Part model, mm, in its own coordinate system. Face numbers are marked on the shaded views. Round coordinates to 2 decimals unless told otherwise and drop trailing zeros. Put each result on its own line as item: value.
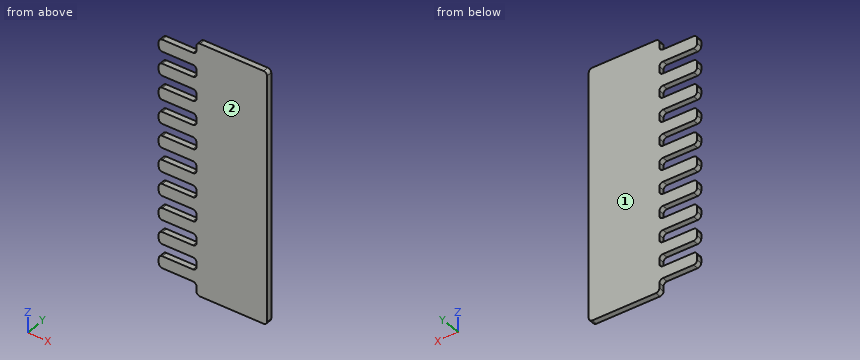
from build123d import *

# Parameters (mm, degrees)
BOSS_EXTRUDE1_DEPTH = 1.2


with BuildPart() as part:
    # Sketch1 → Boss-Extrude1 (new body)
    with BuildSketch(Plane(origin=(0, 0, 0), x_dir=(1, 0, 0), z_dir=(0, 1, 0))):
        with BuildLine():
            Line((-0.75, 2.54), (-7.25, 2.54))
            ThreePointArc((-7.25, 2.54), (-7.780330086, 2.759669914), (-8, 3.29))
            Line((-8, 3.29), (-8, 4.33))
            ThreePointArc((-8, 4.33), (-7.780330086, 4.860330086), (-7.25, 5.08))
            Line((-7.25, 5.08), (-0.75, 5.08))
            ThreePointArc((-0.75, 5.08), (-0.219669914, 5.299669914), (0, 5.83))
            Line((0, 5.83), (0, 6.87))
            ThreePointArc((0, 6.87), (-0.219669914, 7.400330086), (-0.75, 7.62))
            Line((-0.75, 7.62), (-7.25, 7.62))
            ThreePointArc((-7.25, 7.62), (-7.780330086, 7.839669914), (-8, 8.37))
            Line((-8, 8.37), (-8, 9.41))
            ThreePointArc((-8, 9.41), (-7.780330086, 9.940330086), (-7.25, 10.16))
            Line((-7.25, 10.16), (-0.75, 10.16))
            ThreePointArc((-0.75, 10.16), (-0.219669914, 10.379669914), (0, 10.91))
            Line((0, 10.91), (0, 11.95))
            ThreePointArc((0, 11.95), (-0.219669914, 12.480330086), (-0.75, 12.7))
            Line((-0.75, 12.7), (-7.25, 12.7))
            ThreePointArc((-7.25, 12.7), (-7.780330086, 12.919669914), (-8, 13.45))
            Line((-8, 13.45), (-8, 14.49))
            ThreePointArc((-8, 14.49), (-7.780330086, 15.020330086), (-7.25, 15.24))
            Line((-7.25, 15.24), (-0.75, 15.24))
            ThreePointArc((-0.75, 15.24), (-0.219669914, 15.459669914), (0, 15.99))
            Line((0, 15.99), (0, 17.03))
            ThreePointArc((0, 17.03), (-0.219669914, 17.560330086), (-0.75, 17.78))
            Line((-0.75, 17.78), (-7.25, 17.78))
            ThreePointArc((-7.25, 17.78), (-7.780330086, 17.999669914), (-8, 18.53))
            Line((-8, 18.53), (-8, 19.57))
            ThreePointArc((-8, 19.57), (-7.780330086, 20.100330086), (-7.25, 20.32))
            Line((-7.25, 20.32), (-0.75, 20.32))
            ThreePointArc((-0.75, 20.32), (-0.219669914, 20.539669914), (0, 21.07))
            Line((0, 21.07), (0, 22.11))
            ThreePointArc((0, 22.11), (-0.219669914, 22.640330086), (-0.75, 22.86))
            Line((-0.75, 22.86), (-7.25, 22.86))
            ThreePointArc((-7.25, 22.86), (-7.780330086, 23.079669914), (-8, 23.61))
            Line((-8, 23.61), (-8, 24.65))
            ThreePointArc((-8, 24.65), (-7.780330086, 25.180330086), (-7.25, 25.4))
            Line((-7.25, 25.4), (-0.75, 25.4))
            ThreePointArc((-0.75, 25.4), (-0.219669914, 25.619669914), (0, 26.15))
            Line((0, 26.15), (0, 27.19))
            ThreePointArc((0, 27.19), (-0.219669914, 27.720330086), (-0.75, 27.94))
            Line((-0.75, 27.94), (-7.25, 27.94))
            ThreePointArc((-7.25, 27.94), (-7.780330086, 28.159669914), (-8, 28.69))
            Line((-8, 28.69), (-8, 29.73))
            ThreePointArc((-8, 29.73), (-7.780330086, 30.260330086), (-7.25, 30.48))
            Line((-7.25, 30.48), (-0.75, 30.48))
            ThreePointArc((-0.75, 30.48), (-0.219669914, 30.699669914), (0, 31.23))
            Line((0, 31.23), (0, 32.27))
            ThreePointArc((0, 32.27), (-0.219669914, 32.800330086), (-0.75, 33.02))
            Line((-0.75, 33.02), (-7.25, 33.02))
            ThreePointArc((-7.25, 33.02), (-7.780330086, 33.239669914), (-8, 33.77))
            Line((-8, 33.77), (-8, 34.81))
            ThreePointArc((-8, 34.81), (-7.780330086, 35.340330086), (-7.25, 35.56))
            Line((-7.25, 35.56), (-0.75, 35.56))
            ThreePointArc((-0.75, 35.56), (-0.219669914, 35.779669914), (0, 36.31))
            Line((0, 36.31), (0, 37.35))
            ThreePointArc((0, 37.35), (-0.219669914, 37.880330086), (-0.75, 38.1))
            Line((-0.75, 38.1), (-7.25, 38.1))
            ThreePointArc((-7.25, 38.1), (-7.780330086, 38.319669914), (-8, 38.85))
            Line((-8, 38.85), (-8, 39.89))
            ThreePointArc((-8, 39.89), (-7.780330086, 40.420330086), (-7.25, 40.64))
            Line((-7.25, 40.64), (-0.75, 40.64))
            ThreePointArc((-0.75, 40.64), (-0.219669914, 40.859669914), (0, 41.39))
            Line((0, 41.39), (0, 42.43))
            ThreePointArc((0, 42.43), (-0.219669914, 42.960330086), (-0.75, 43.18))
            Line((-0.75, 43.18), (-7.25, 43.18))
            ThreePointArc((-7.25, 43.18), (-7.780330086, 43.399669914), (-8, 43.93))
            Line((-8, 43.93), (-8, 44.97))
            ThreePointArc((-8, 44.97), (-7.780330086, 45.500330086), (-7.25, 45.72))
            Line((-7.25, 45.72), (-0.75, 45.72))
            ThreePointArc((-0.75, 45.72), (-0.219669914, 45.939669914), (0, 46.47))
            Line((0, 46.47), (0, 47.51))
            ThreePointArc((0, 47.51), (-0.219669914, 48.040330086), (-0.75, 48.26))
            Line((-0.75, 48.26), (-7.25, 48.26))
            ThreePointArc((-7.25, 48.26), (-7.780330086, 48.479669914), (-8, 49.01))
            Line((-8, 49.01), (-8, 50.05))
            ThreePointArc((-8, 50.05), (-7.780330086, 50.580330086), (-7.25, 50.8))
            Line((-7.25, 50.8), (-0.75, 50.8))
            ThreePointArc((-0.75, 50.8), (-0.219669914, 51.019669914), (0, 51.55))
            Line((0, 51.55), (0, 52.59))
            ThreePointArc((0, 52.59), (0.219669914, 53.120330086), (0.75, 53.34))
            Line((0.75, 53.34), (14.25, 53.34))
            ThreePointArc((14.25, 53.34), (14.780330086, 53.120330086), (15, 52.59))
            Line((15, 52.59), (15, 0.75))
            ThreePointArc((15, 0.75), (14.780330086, 0.219669914), (14.25, 0))
            Line((14.25, 0), (0.75, 0))
            ThreePointArc((0.75, 0), (0.219669914, 0.219669914), (0, 0.75))
            Line((0, 0.75), (0, 1.79))
            ThreePointArc((0, 1.79), (-0.219669914, 2.320330086), (-0.75, 2.54))
        make_face()
    extrude(amount=BOSS_EXTRUDE1_DEPTH)


solid = part.part
1. Pin check, flat tips, straight feed: P1, Ø0.5, axis at y = 0.5, z = -1.5, coming from the -X side; P2, Ø0.6, axis at x = -3.5, y = 0.5, coming from the -Z side. Stop position of each tip, or through.
A:
P1: stops at x = 0
P2: stops at z = -50.8
2. Band-saw the part on A-A (x = -3.5). Give the number of separate pieces and of enclosed holes in the cut face, plus the area to 3 significant figures.
A:
separate pieces: 10
enclosed holes: 0
area: 30.5 mm²
3. Two-plate mould, pull along Y, no slides. Class the marked faces 1 and 2: pulls with the +Y half, pulls with the -Y half, needs draft (parallel to the pull), parting line crosses it, or undercut.
A:
face 1: pulls with the +Y half
face 2: pulls with the -Y half
4. Probe line 1 along X through (y, z) = (0.2, -41.5); line 2 along X through (y, z) = (0.9, -5). List the from-to ranges inside material, lowest first. Write a range as [from, to].
A:
line 1: x = [0, 15]
line 2: x = [-7.59, 15]
